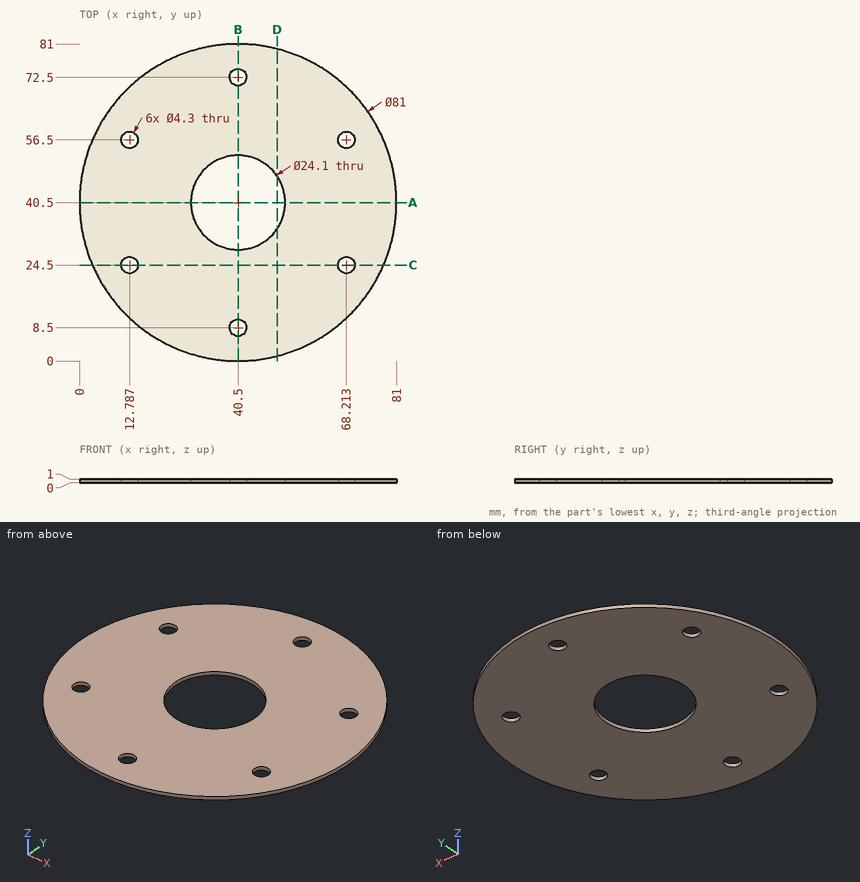
Print and shaded views of the part. All mm, measured from the part's lowest x, y and z. Round coordinates to 2 decimals unless told otherwise and drop trailing zeros. Write each loop counter-clockwise with the first axis right and the second up, starting at its lowest first coordinate (ties: lowest second). Pieces come first, ordered by that corner, then holes.
(1) Drop a flat-ended pin along its axis: P1, Ø4, axis at x = 40.5, y = 72.5, coming from the +Z side. Give the stop position or say it passes through.
(2) Slice it at A-A, the plane y = 40.5. Write the cut outline in (x, z).
(3) Slice it at C-C, the plane y = 24.5. Write the cut outline in (x, z).
(4) Slice it at B-B, the plane x = 40.5. Write the cut outline in (y, z).
(5) Probe line 1 along Y through (x, z) = (40.5, 0.4); line 2 along X through (y, z) = (25.5, 0.5); line 3 along X through (y, z) = (24.5, 0.5) (1 decimal). List the from-to ranges inside material, lowest first.
(6) Slice it at D-D, the plane x = 50.5. Write the cut outline in (y, z).
From the geometry:
1. P1: passes through
2. outline: (0, 0) - (28.45, 0) - (28.45, 1) - (0, 1) - close; (52.55, 0) - (81, 0) - (81, 1) - (52.55, 1) - close
3. outline: (3.29, 0) - (10.64, 0) - (10.64, 1) - (3.29, 1) - close; (14.94, 0) - (66.06, 0) - (66.06, 1) - (14.94, 1) - close; (70.36, 0) - (77.71, 0) - (77.71, 1) - (70.36, 1) - close
4. outline: (0, 0) - (6.35, 0) - (6.35, 1) - (0, 1) - close; (10.65, 0) - (28.45, 0) - (28.45, 1) - (10.65, 1) - close; (52.55, 0) - (70.35, 0) - (70.35, 1) - (52.55, 1) - close; (74.65, 0) - (81, 0) - (81, 1) - (74.65, 1) - close
5. line 1: y = 0 to 6.35, 10.65 to 28.45, 52.55 to 70.35, 74.65 to 81
5. line 2: x = 2.88 to 10.88, 14.69 to 66.31, 70.12 to 78.12
5. line 3: x = 3.3 to 10.6, 14.9 to 66.1, 70.4 to 77.7
6. outline: (1.25, 0) - (33.78, 0) - (33.78, 1) - (1.25, 1) - close; (47.22, 0) - (79.75, 0) - (79.75, 1) - (47.22, 1) - close
